Model file for the job. Use its own axes, mm. Give positions to 0.01 mm unless a question says otherwise; leave off trailing zeros. Write each loop counter-clockwise with the first axis right and the second up, starting at its lowest first coordinate (ties: lowest second). Pieces come first, ordered by that corner, then holes.
```python
from build123d import *

# Parameters (mm, degrees)
F0_R     = 1.621513
F0_R_2   = 1.620764
F0_W     = 260.302752
F0_H     = 116.467979
F0_R_3   = 1.624073
F0_R_4   = 1.618261
F1_DEPTH = 15


with BuildPart() as f1:
    # F0 (on Top) → F1 (new body)
    with BuildSketch(Plane.XY):
        Polygon((138.743147, 67.134982), (138.351147, 67.149982), (-138.350253, 67.150982), (-138.742993, 67.134982), (-139.132953, 67.088982), (-139.517453, 67.011982), (-139.896403, 66.905982), (-140.264343, 66.768982), (-140.619873, 66.604982), (-140.963003, 66.413982), (-141.289603, 66.195982), (-141.598283, 65.953982), (-141.886293, 65.685982), (-142.153633, 65.398982), (-142.396163, 65.089982), (-142.613896, 64.762982), (-142.805443, 64.419982), (-142.969429, 64.063982), (-143.105855, 63.695982), (-143.211965, 63.317982), (-143.289135, 62.932982), (-143.33461, 62.542982), (-143.349768, 62.149982), (-143.351146, -62.150088), (-143.33461, -62.542838), (-143.289135, -62.932798), (-143.211965, -63.317288), (-143.105855, -63.696238), (-142.969429, -64.064178), (-142.805443, -64.419708), (-142.613896, -64.762838), (-142.396163, -65.089438), (-142.153633, -65.398118), (-141.886293, -65.686128), (-141.598283, -65.953468), (-141.289603, -66.195998), (-140.963003, -66.41373), (-140.619873, -66.605278), (-140.264343, -66.769266), (-139.896403, -66.905691), (-139.517453, -67.0118), (-139.132953, -67.08897), (-138.742993, -67.134446), (-138.350253, -67.150982), (138.351147, -67.150982), (138.743147, -67.134446), (139.133147, -67.08897), (139.517147, -67.0118), (139.896147, -66.905691), (140.264147, -66.769266), (140.620147, -66.605278), (140.963147, -66.41373), (141.289147, -66.195998), (141.598147, -65.953468), (141.886147, -65.686128), (142.153147, -65.398118), (142.396147, -65.089438), (142.614147, -64.762838), (142.805147, -64.419708), (142.969147, -64.064178), (143.106147, -63.696238), (143.212147, -63.317288), (143.289147, -62.932798), (143.334147, -62.542838), (143.351147, -62.151458), (143.350147, 62.149982), (143.334147, 62.542982), (143.289147, 62.932982), (143.212147, 63.317982), (143.106147, 63.695982), (142.969147, 64.063982), (142.805147, 64.419982), (142.614147, 64.762982), (142.396147, 65.089982), (142.153147, 65.398982), (141.886147, 65.685982), (141.598147, 65.953982), (141.289147, 66.195982), (140.963147, 66.413982), (140.620147, 66.604982), (140.264147, 66.768982), (139.896147, 66.905982), (139.517147, 67.011982), (139.133147, 67.088982), align=None)
        with Locations((-138.351685, -62.138656)):
            Circle(F0_R, mode=Mode.SUBTRACT)
        with Locations((138.346991, -62.147275)):
            Circle(F0_R_2, mode=Mode.SUBTRACT)
        with Locations((-0.470817, 0.892164)):
            Rectangle(F0_W, F0_H, mode=Mode.SUBTRACT)
        with Locations((-138.354012, 62.161052)):
            Circle(F0_R_3, mode=Mode.SUBTRACT)
        with Locations((138.34434, 62.144211)):
            Circle(F0_R_4, mode=Mode.SUBTRACT)
    extrude(amount=F1_DEPTH)


solid = f1.part
```
1. Slice it at A-A, the plane y = -2. Write the cut outline in (x, z), and give its area (3 significant figures).
Calculated:
outline: (-143.35, 0) - (-130.62, 0) - (-130.62, 15) - (-143.35, 15) - close; (129.68, 0) - (143.35, 0) - (143.35, 15) - (129.68, 15) - close
area: 396 mm2
2. Slice it at C-C, the plane z = 7.75. State how many separate pieces and enclosed holes the cut face has, and give its area (3 significant figures).
Calculated:
separate pieces: 1
enclosed holes: 5
area: 8,130 mm2
3. Probe probe 1 along X at (y, z) = (-6.5, 4.75); probe 2 along Y at (x, z) = (-38, 7). List the from-to ranges inside material, lowest first.
Calculated:
probe 1: x = -143.35 to -130.62, 129.68 to 143.35
probe 2: y = -67.15 to -57.34, 59.13 to 67.15
4. Slice it at B-B, the plane x = -8.5. Write the cut outline in (y, z), and give its area (3 significant figures).
Calculated:
outline: (-67.15, 0) - (-57.34, 0) - (-57.34, 15) - (-67.15, 15) - close; (59.13, 0) - (67.15, 0) - (67.15, 15) - (59.13, 15) - close
area: 268 mm2
5. Pull direction Z, two halves, no side cores. Call faces 1 (the flat face through (-11, -59, 15)), 2 (the flat face through (-11, -59, 0)), 3 (the flat face through (-2, -67.151, 7)): +Z half, -Z half, draft (parallel to the pull), parting line (faces both ways), or undercut.
Calculated:
face 1: +Z half
face 2: -Z half
face 3: draft
